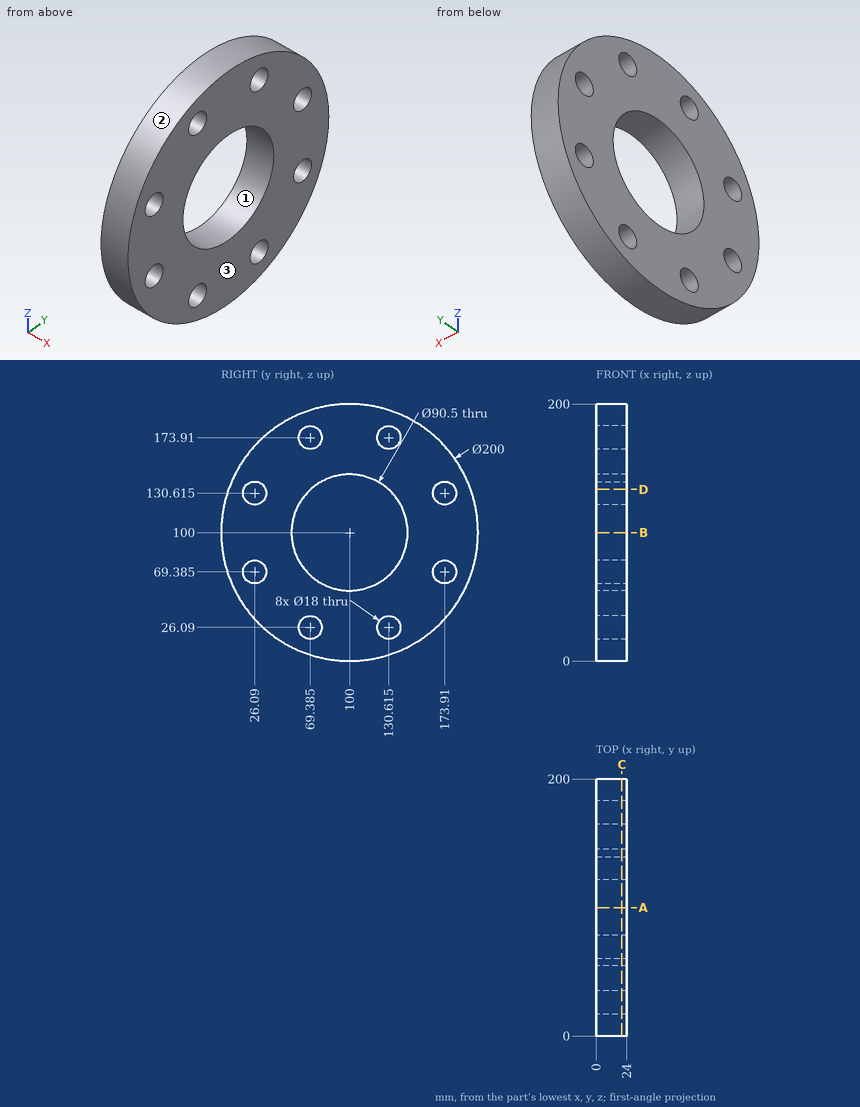
Source: three-view drawing plus pictorial views. Frame: mm from the lowest corner of the part. Give positions to 0.01 mm unless a question says otherwise; leave off trailing zeros. Write each loop counter-clockwise with the first axis right and the second up, starting at its lowest first coordinate (ties: lowest second). Pieces come first, ordered by that corner, then holes. Notation, with made-up numbers: (12.25, -5.75) - (56.25, -5.75) arc R28 ccw to (56.25, 13.25) - close; hole circle Ø11 at (85.5, 71.5). An arc over 180 degrees is marked (long way). Write item = value, one per line. Start each with the question number.
1. Ray query, L1, parallel to Z at x = 21, y = 172.5 (1 decimal); L2, parallel to Z at x = 8.25, y = 170.5 (1 decimal); L3, parallel to Z at x = 9.75, y = 100. Return the intervals inside material, ascending.
2. First-contact query: pin 1 Ø14.5 at (y, z) = (69.39, 26.09) entering from +X; pin 2 Ø1 at (x, z) = (16.5, 71) entering from -Y; pin 3 Ø4 at (x, y) = (21.5, 168.5) entering from +Z (1 decimal); pin 4 Ø1.5 at (x, z) = (14.5, 33.5) entering from +Y (1 decimal). Flat tips, straight axial feed; report the tip coordinate or a pass-through.
3. Section query C-C, the plane x = 20. Count the separate pieces of the cut face and the enclosed holes in it, then the cut area to 3 significant figures.
4. Section query D-D, the plane z = 133.5. Output: boundary loops of the cut face in (x, y) (1 decimal), then the cut area to 3 significant figures.
5. Section query A-A, the plane y = 100. Output: boundary loops of the cut face in (x, z), then the cut area to 3 significant figures.
6. Mould query, pull axis Z, two halves, no side actions, for the marked faces 1, 2 and 3. Classes: released by +Z, released by -Z, zero draft, split by the parting line, or undercut.
Check sheet entries:
q1.L1 = 31.1 to 60.5, 78.3 to 121.7, 139.5 to 168.9
q1.L2 = 29.1 to 61.1, 77.7 to 122.3, 138.9 to 170.9
q1.L3 = 0 to 54.75, 145.25 to 200
q2.pin_1 = through
q2.pin_2 = 4.15
q2.pin_3 = 174.7
q2.pin_4 = 175.3
q3.separate_pieces = 1
q3.enclosed_holes = 9
q3.area = 22,900 mm2
q4.outline = (0, 5.8) - (24, 5.8) - (24, 17.6) - (0, 17.6) - close; (0, 34.6) - (24, 34.6) - (24, 69.6) - (0, 69.6) - close; (0, 130.4) - (24, 130.4) - (24, 165.4) - (0, 165.4) - close; (0, 182.4) - (24, 182.4) - (24, 194.2) - (0, 194.2) - close
q4.area = 2,240 mm2
q5.outline = (0, 0) - (24, 0) - (24, 54.75) - (0, 54.75) - close; (0, 145.25) - (24, 145.25) - (24, 200) - (0, 200) - close
q5.area = 2,630 mm2
q6.face_1 = undercut
q6.face_2 = split by the parting line
q6.face_3 = zero draft
